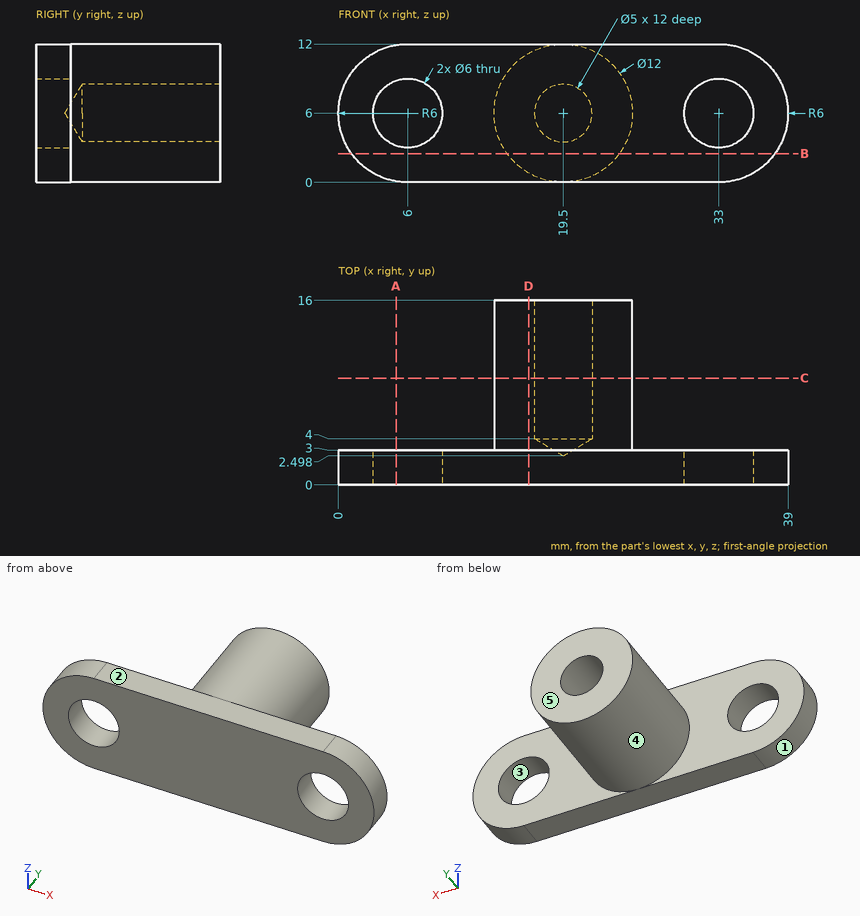
Design review of the part shown in the three views and the two pictorial views. Dimensions are in mm from the part's minimum x, y and z. A direction names the side the tool comes from. Coordinates: 2 decimals unless noted, no trailing zeros. Order: outer loops, then holes, each group sorted by start corner. A loop starts at its lowest first (then second) coordinate and runs counter-clockwise, first axis right, second up. Notation, with made-up numbers: (14.5, 83.5) -> (37.5, 83.5) arc R8 cw to (37.5, 94.5) -> close; hole circle Ø3 at (57, 62.5). An arc over 180 degrees is marked (long way). Use one line per item in the form item = value. Start each with the question number.
(1) Add section C-C on y = 9.25. State the section outline as (x, z) points.
(2) The part is to be moulded in two halves that separate along X. For the marked faces 1, 2 and 3, say which applies: +X half, -X half, draft (parallel to the pull), parting line (faces both ways), or undercut.
(3) Insertion check: pin 1 (1 mm diameter, centred on y = 14, z = 10.5, fed in from -X); pin 2 (4 mm diameter, centred on y = 9, z = 4.5, fed in from +X); pin 3 (6 mm diameter, centred on x = 19.5, z = 6, fed in from +Y); pin 4 (4 mm diameter, centred on x = 16, y = 5.5, fed in from -Z). Each pin has a flat end and moves straight along its axis. Give the tip position at first contact, or say it passes through.
(4) For the marked faces 4 and 5, list the 3-axis set-ups (+Z, -Z, +X, -X, +Y, -Y) from which the entire face can be reached by the end or side of a thin tool; tool diameter is ignored.
(5) Add section B-B on z = 2.5. State the section outline as (x, y) points, plus the area to 3 significant figures.
(6) Add section A-A on x = 5. State the section outline as (y, z) points.
(7) For probe 1 along Z at (x, y) = (19.5, 8.5); probe 2 along X at (y, z) = (1.25, 6); probe 3 along Y at (x, z) = (10.5, 10.5), list the stretches that pass through material, from the lowest coordinate up.
(8) Add section D-D on x = 16.5. State the section outline as (y, z) points.
Answer block:
q1.outline = circle Ø12 at (19.5, 6); hole circle Ø5 at (19.5, 6)
q2.face_1 = -X half
q2.face_2 = draft
q2.face_3 = undercut
q3.pin_1 = 15.03
q3.pin_2 = 25.5
q3.pin_3 = 16
q3.pin_4 = 0.19
q4.face_4 = +Y
q4.face_5 = +Z, -Z, +X, -X, +Y
q5.outline = (1.13, 0) -> (37.87, 0) -> (37.87, 3) -> (24.37, 3) -> (24.37, 16) -> (14.63, 16) -> (14.63, 3) -> (1.13, 3) -> close
q5.area = 237 mm²
q6.outline = (0, 0.08) -> (3, 0.08) -> (3, 3.17) -> (0, 3.17) -> close; (0, 8.83) -> (3, 8.83) -> (3, 11.92) -> (0, 11.92) -> close
q7.probe_1 = 0 to 3.5, 8.5 to 12
q7.probe_2 = 0 to 3, 9 to 30, 36 to 39
q7.probe_3 = 0 to 3
q8.outline = (0, 0) -> (3, 0) -> (3, 0.8) -> (16, 0.8) -> (16, 11.2) -> (3, 11.2) -> (3, 12) -> (0, 12) -> close
